Can you work these out from the model? Positions are in its coordinate system, mm. A direction names the side the tool comes from. Round coordinates to 2 decimals unless told otherwise and drop trailing zeros. Loops run counter-clockwise (first coordinate to the right, second up) from the corner with the lowest first, then second, coordinate; pieces in that order, holes last. Notation, with made-up numbers: M -20.5,8.25 L -0.5,8.25 A11 cw -0.5,27.25 Z; hole C 6,86.25 d1. An arc over 180 degrees is marked long. Return JSON: item names as keys, results as strings.
Autodesk Inventor part; units mm, degrees
ref_plane "YZ Plane" through (0, 0, 0) normal (1, 0, 0) x (0, 1, 0)
ref_plane "XZ Plane" through (0, 0, 0) normal (0, 1, 0) x (-1, 0, 0)
ref_plane "XY Plane" through (0, 0, 0) normal (0, 0, 1) x (1, 0, 0)
sketch "草圖2" plane through (0, 0, 0) normal (0, 1, 0) x (-1, 0, 0)
  line L0 (0, 0) -> (10, 0)
  line L1 (10, 0) -> (10, -20)
  line L2 (10, -20) -> (0, -20)
  line L3 (0, -20) -> (0, 0)
  dimension "d1" = 10
  dimension "d2" = 20
extrude "擠出1" add sketch "草圖2" along normal blind 3
fillet "圓角1" radius 1 4 edges at (-10, 3, -10) (0, 3, -10) (0, 0, -10) (-10, 0, -10)
sketch "草圖3" plane through (-9, 0, 0) normal (0, 0, 1) x (1, 0, 0)
  line L0 (1.3959, 0.8511) -> (6.3959, 0.8511)
  line L1 (6.3959, 0.8511) -> (6.3959, 2.1511)
  line L2 (6.3959, 2.1511) -> (1.3959, 2.1511)
  line L3 (1.3959, 2.1511) -> (1.3959, 0.8511)
  point P0 (9, 0)
  dimension "d6" = 5
  dimension "d7" = 1.3
extrude "擠出2" add sketch "草圖3" along normal blind 6
sketch "草圖4" plane through (-9, 0, 6) normal (0, 0, 1) x (1, 0, 0)
  line L0 (6.0686, 1.499) -> (1.5686, 1.499)
  line L1 (1.5686, 1.499) -> (1.5686, 0.999)
  line L2 (1.5686, 0.999) -> (6.0686, 0.999)
  line L3 (6.0686, 0.999) -> (6.0686, 1.499)
  line L4 (4.9801, 1.499) -> (4.9403, 1.499)
  point P0 (9, 0)
  dimension "d12" = 4.5
  dimension "d13" = 0.5
extrude "擠出3" cut sketch "草圖4" against normal blind 6
properties part number "USB"
Q1. If I drill on line 1 along X through (y, z) = (1.45, 1.25); line 2 along Z through (x, y) = (-4.5, 0.3); line 3 along Y through (x, z) = (-9.5, -5.25), over which ranges is the centre line in solid material (lowest first)?
Results:
{"line 1": "x = -7.6 to -7.43, -2.93 to -2.6", "line 2": "z = -20 to 0", "line 3": "y = 0.13 to 2.87"}
Q2. Suppose I cut it at B-B, the plane x = -4.5. Please give me the cut outline in (y, z).
Results:
{"outline": "M 0,-20 L 3,-20 L 3,0 L 2.15,0 L 2.15,6 L 1.5,6 L 1.5,0 L 1,0 L 1,6 L 0.85,6 L 0.85,0 L 0,0 Z"}
Q3. Thinking about a two-plate mould opening in Y: for faces 4 (the flat face through (-7.604, 2, 3)), 5 (the flat face through (-5, 1.499, 3)), 6 (the cylindrical face through (-9.699, 0.285, -10.14)), which applies, pulls with the +Y half, pulls with the -Y half, needs draft (parallel to the pull), parting line crosses it, or undercut?
Results:
{"face 4": "needs draft", "face 5": "undercut", "face 6": "pulls with the -Y half"}
Q4. On a 3-axis mill with a long thin cutter (end or side, diameter ignored), from which of +Z, -Z, +X, -X, +Y, -Y can I reach the whole of each face in a straight line? I mean faces 1 (the cylindrical face through (-9.715, 2.699, -10.14)), 2 (the flat face through (-5, 2.151, 3)), 3 (the flat face through (-2.604, 1.5, 3)). Say none if no direction works.
Results:
{"face 1": "+Z, -Z, -X, +Y", "face 2": "+Z, +X, -X, +Y", "face 3": "+Z, +X, +Y, -Y"}
Q5. Suppose I cut it at A-A, the plane z = -2. Please give me the cut outline in (x, y).
Results:
{"outline": "M -10,1 A1 ccw -9,0 L -1,0 A1 ccw 0,1 L 0,2 A1 ccw -1,3 L -9,3 A1 ccw -10,2 Z"}
Q6. I'm going to push flat-ended pins straight in: pin 1 Ø0.6 at (y, z) = (1, 3) entering from -X; pin 2 Ø5 at (x, z) = (-5, 4) entering from +Y; pin 3 Ø4 at (x, z) = (-7.5, -15.5) entering from -Y; pin 4 Ø4 at (x, z) = (-5.5, 4) entering from -Y. Where does each tip first touch, or does it pass through?
Results:
{"pin 1": "stops at x = -7.6", "pin 2": "stops at y = 2.15", "pin 3": "stops at y = 0", "pin 4": "stops at y = 0.85"}
Q7. Suppose I cut it at D-D, the plane x = -8.75. Please give me the cut outline in (y, z), plus the area to 3 significant figures.
Results:
{"outline": "M 0,-20 L 3,-20 L 3,0 L 0,0 Z", "area": "60.0 mm2"}
Q8. Suppose I cut it at C-C, the plane y = 0.5. Please give me the cut outline in (x, z).
Results:
{"outline": "M -9.87,-20 L -0.13,-20 L -0.13,0 L -9.87,0 Z"}
